```python
from build123d import *

# Parameters (mm, degrees)
SKETCH2_R            = 50
BOSS_EXTRUDE1_DEPTH  = 150
SKETCH3_OUTSIDE_W    = 143.232
SKETCH3_OUTSIDE_H    = 143.232
CUT_EXTRUDE1_DEPTH   = 120
CUT_SWEEP1_PROFILE_R = 10


with BuildPart() as part:
    # Sketch2 → Boss-Extrude1 (new body)
    with BuildSketch(Plane.XY):
        Circle(SKETCH2_R)
    extrude(amount=BOSS_EXTRUDE1_DEPTH)

    # Sketch3 outside → Cut-Extrude1 (cut)
    with BuildSketch(Plane.XY.offset(150)):
        Rectangle(SKETCH3_OUTSIDE_W, SKETCH3_OUTSIDE_H)
        with BuildLine():
            Line((-45.82575695, 20), (45.82575695, 20))
            ThreePointArc((45.82575695, 20), (0, 50), (-45.82575695, 20))
        make_face(mode=Mode.SUBTRACT)
        with BuildLine():
            Line((45.82575695, -20), (-45.82575695, -20))
            ThreePointArc((-45.82575695, -20), (0, -50), (45.82575695, -20))
        make_face(mode=Mode.SUBTRACT)
    extrude(amount=-CUT_EXTRUDE1_DEPTH, mode=Mode.SUBTRACT)

    # Cut-Sweep1: sweep along a path in Sketch5
    with BuildLine(Plane.XY.offset(90)) as cut_sweep1_path:
        Line((0, 50), (0, -50))
    # Cut-Sweep1 profile (on start of the path) → Cut-Sweep1 (sweep, cut)
    with BuildSketch(Plane(origin=(0, 50, 90), x_dir=(-1, 0, 0), z_dir=(0, -1, 0))):
        Circle(CUT_SWEEP1_PROFILE_R)
    sweep(path=cut_sweep1_path.line, mode=Mode.SUBTRACT)


solid = part.part
```
The listing builds one solid part. Answer for the finished solid, in the listing's coordinates (mm). A direction names the side the tool comes from. Give positions to 0.01 mm unless a question says otherwise; leave off trailing zeros. Loops run counter-clockwise (first coordinate to the right, second up) from the corner with the lowest first, then second, coordinate; pieces in that order, holes last. Notation, with made-up numbers: (67.25, -37.5) - (124.25, -37.5) arc R17 cw to (124.25, -14.5) - close; hole circle Ø10 at (61.5, -15.75). An arc over 180 degrees is marked (long way). Return JSON: item names as keys, results as strings. Group by question number.
1. Given pin 1 Ø10 at (x, z) = (35.5, 43.5) entering from -Y; pin 2 Ø10 at (y, z) = (-21.5, 77.5) entering from +X; pin 3 Ø10 at (x, z) = (-16, 77.5) entering from -Y (3 decimals); pin 4 Ø6 at (x, y) = (34, -38) entering from +Z, each flat-ended and moving along its own axis, determine where each tip first touches the part or whether it passes through.
2. Straight lines are drawn through the part: line 1 (Z direction, x = 0, y = 41); line 2 (Y direction, x = -7.5, z = 63); line 3 (Y direction, x = 10, z = 79). For each, find the intervals that lie inside material, in ascending order. Write a range as [from, to].
3. Which of the six approach directions +Z, -Z, +X, -X, +Y, -Y give full straight-line access (tool end or side, diameter ignored) to faces 1 (the flat face through (11, -20, 91)), 2 (the flat face through (-1, 1, 0))?
4. Find section D-D (y = 25). Write down the section's boundary in (x, z), then the cut area to 3 significant figures.
5. Find section A-A (x = 0). Write down the section's boundary in (y, z).
6. Determine the mould class of faces 3 (the flat face through (-11, 20, 91)), 4 (the cylindrical face through (1.302, 34.79, 80.085)), 5 (the cylindrical face through (-40, -30, 74)) for opening direction X: pulls with the +X half, pulls with the -X half, needs draft (parallel to the pull), parting line crosses it, or undercut.
7. Find section C-C (z = 59). Write down the section's boundary in (x, y).
8. Find section B-B (z = 90). Write down the section's boundary in (x, y), then the cut area to 3 significant figures.
Verdict:
{
 "1": {"pin 1": "stops at y = -39.62", "pin 2": "stops at x = 45.83", "pin 3": "stops at y = -48.775", "pin 4": "stops at z = 150"},
 "2": {"line 1": "z = [0, 80], [100, 150]", "line 2": "y = [-49.43, -20], [20, 49.43]", "line 3": "y = [-48.99, -20], [20, 48.99]"},
 "3": {"face 1": "+Z, +X, -X", "face 2": "-Z, +X, -X, +Y, -Y"},
 "4": {"outline": "(-43.3, 0) - (43.3, 0) - (43.3, 150) - (-43.3, 150) - close; hole circle Ø20 at (0, 90)", "area": "12,700 mm^2"},
 "5": {"outline": "(-50, 0) - (50, 0) - (50, 80) - (20, 80) - (20, 30) - (-20, 30) - (-20, 80) - (-50, 80) - close; (-50, 100) - (-20, 100) - (-20, 150) - (-50, 150) - close; (20, 100) - (50, 100) - (50, 150) - (20, 150) - close"},
 "6": {"face 3": "needs draft", "face 4": "undercut", "face 5": "parting line crosses it"},
 "7": {"outline": "(-45.83, -20) arc R50 ccw to (45.83, -20) - close; (-45.83, 20) - (45.83, 20) arc R50 ccw to start"},
 "8": {"outline": "(-45.83, -20) arc R50 ccw to (-10, -48.99) - (-10, -20) - close; (-45.83, 20) - (-10, 20) - (-10, 48.99) arc R50 ccw to start; (10, -48.99) arc R50 ccw to (45.83, -20) - (10, -20) - close; (10, 20) - (45.83, 20) arc R50 ccw to (10, 48.99) - close", "area": "2,780 mm^2"}
}
